```python
from build123d import *

# Parameters (mm, degrees)
F0_R     = 1.5
F2_DEPTH = 50
F3_DEPTH = 60
F4_W     = 40
F4_H     = 40
F5_DEPTH = 140.1
F6_R     = 17.5
F7_DEPTH = 25.001


with BuildPart() as f2:
    # F0 (on Top) → F2 (new body)
    with BuildSketch(Plane.XY):
        with BuildLine():
            Line((150.375, 22.496875), (0.416667, 24.996528))
            ThreePointArc((0.416667, 24.996528), (-25, 0), (0.416667, -24.996528))
            Line((0.416667, -24.996528), (150.375, -22.496875))
            ThreePointArc((150.375, -22.496875), (172.5, 0), (150.375, 22.496875))
        make_face()
        with Locations((150, 0)):
            Circle(F0_R, mode=Mode.SUBTRACT)
    extrude(amount=F2_DEPTH)

    # F1 (on face) → F3 (cut)
    with BuildSketch(Plane.XY):
        Polygon((5, 10.392305), (5, -10.392305), (23, -20.784609), (41, -10.392305), (41, 10.392305), (23, 20.78461), align=None)
        Polygon((82, -10.392305), (82, 10.392305), (64, 20.78461), (46, 10.392305), (46, -10.392305), (64, -20.784609), align=None)
        Polygon((87, 10.392305), (87, -10.392305), (105, -20.784609), (123, -10.392305), (123, 10.392305), (105, 20.78461), align=None)
    extrude(amount=F3_DEPTH, mode=Mode.SUBTRACT)

    # F4 (on Right) → F5 (cut)
    with BuildSketch(Plane.YZ):
        with Locations((0, 25)):
            Rectangle(F4_W, F4_H)
    extrude(amount=F5_DEPTH, mode=Mode.SUBTRACT)

    # F6 (on Right) → F7 (cut, through all)
    with BuildSketch(Plane.YZ):
        with Locations((0, 25)):
            Circle(F6_R)
    extrude(amount=-F7_DEPTH, mode=Mode.SUBTRACT)


solid = f2.part
```
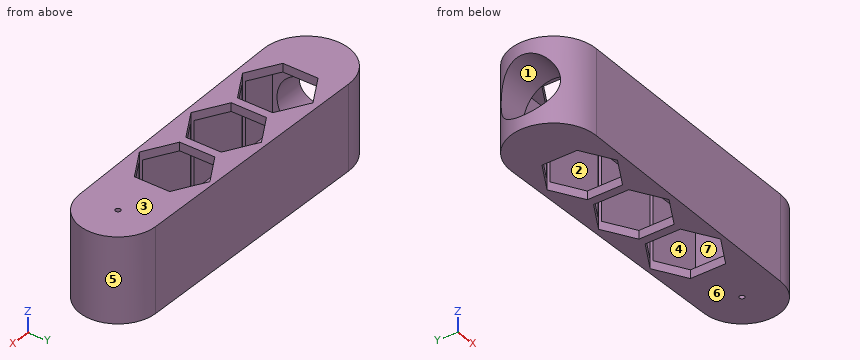
Source: CAD feature listing. Evaluate the final solid. Frame: model axes, mm. Face numbers are marked on the shaded views. A direction names the side the tool comes from. Round coordinates to 2 decimals unless told otherwise and drop trailing zeros. Write each loop counter-clockwise with the first axis right and the second up, starting at its lowest first coordinate (ties: lowest second). Pieces come first, ordered by that corner, then holes. Notation, with made-up numbers: M -29.5,87.5 L -25.5,87.5 A22 cw -25.5,99.5 Z; hole C 87,-14.75 d4. An arc over 180 degrees is marked long. Use CSV: the item, a comma, the result in double quotes. Start each with the question number.
Q1. First-contact query: P1, Ø6, axis at x = 58, z = 24.5, coming from the -Y side; P2, Ø4, axis at y = 4.5, z = 47, coming from the +X side; P3, Ø2.5, axis at y = -5, z = 1.5, coming from the +X side. Flat tips, straight axial feed; report the tip coordinate or a pass-through.
Q2. Line query: line 1 (Z direction, x = 1.5, y = -7.5); line 2 (Y direction, x = 120.5, z = 9); line 3 (X direction, y = 6.5, z = 7.5). Output: solid intervals per line, ascending. Write a range as from..to.
Q3. Cut plane D-D on y = -13. Count the separate pieces of the cut face and the enclosed holes in it, plus the area to 3 significant figures.
Q4. Access query for the marked faces 1, 2 and 3. Directions: +Z, -Z, +X, -X, +Y, -Y. A direction counts if a zero-diameter tool reaches every point of the face in a straight line with its end or side. Return the directions, or none.
Q5. Pull-direction query (Z, two-part tool) for the marked faces 4, 5, 6 and 7; classes: +Z half, -Z half, draft (parallel to the pull), parting line (faces both ways), or undercut.
Q6. Cut plane C-C on x = -8. Output: boundary loops of the cut face in (y, z), plus the area to 3 significant figures.
Q7. Cut plane A-A on x = 19. Output: boundary loops of the cut face in (y, z).
Results found:
1,P1,"y = -24.09"
1,P2,"x = 172.36"
1,P3,"x = 172.19"
2,line 1,"0..5, 45..50"
2,line 2,"-22.99..-20, 20..22.99"
2,line 3,"-24.14..0, 140.1..171.54"
3,separate pieces,"7"
3,enclosed holes,"0"
3,area,"2,570 mm^2"
4,face 1,"-X"
4,face 2,"none"
4,face 3,"+Z, +X, -X, +Y, -Y"
5,face 4,"undercut"
5,face 5,"draft"
5,face 6,"-Z half"
5,face 7,"undercut"
6,outline,"M -23.69,0 L 23.69,0 L 23.69,50 L -23.69,50 Z; hole C 0,25 d35"
6,area,"1,410 mm^2"
7,outline,"M -24.69,0 L -18.48,0 L -18.48,5 L -20,5 L -20,45 L -18.48,45 L -18.48,50 L -24.69,50 Z; M 18.48,0 L 24.69,0 L 24.69,50 L 18.48,50 L 18.48,45 L 20,45 L 20,5 L 18.48,5 Z"
